Geometry: final body of the model. Coordinates: model frame, mm. A direction names the side the tool comes from. Give positions to 0.01 mm unless a question says otherwise; leave off trailing zeros. Order: outer loops, then holes, each group sorted by start corner. A loop starts at its lowest first (then second) coordinate and runs counter-clockwise, first axis right, second up. Notation, with made-up numbers: (-33, 63) - (-22, 63) arc R19 ccw to (-22, 68) - close; hole circle Ø4 at (-18.75, 35.25). An arc over 180 degrees is marked (long way). Put each result on its own line as item: value. Start each with the question number.
1. Mould query, pull axis Y, two halves, no side actions, for faces 1 (the flat face through (878.439, -338, 10)), 2 (the flat face through (672, -459.74, 10)), 3 (the flat face through (679, -254, 20.32)). Classes: pulls with the +Y half, pulls with the -Y half, needs draft (parallel to the pull), parting line crosses it, or undercut.
2. First-contact query: P1, Ø6, axis at x = 509, z = 14, coming from the +Y side. Flat tip, straight axial feed; report the tip coordinate or a pass-through.
3. Section C-C on x = 664.5. Return the cut outline in (y, z), plus the area to 3 significant figures.
4. Section B-B on z = 6. Count the separate pieces of the cut face and the enclosed holes in it, plus the area to 3 significant figures.
5. Set-up query: faces 4 (the flat face through (348, -44.45, 10)), 5 (the flat face through (508, -459.74, 10)), 6 (the flat face through (508, -54.61, 10)), 7 (the flat face through (878.439, -176, 10)), 8 (the flat face through (348, -469.9, 10)). Return all of +Z, -Z, +X, -X, +Y, -Y with unobstructed straight access to the full face (end or side cutting, diameter ignored); none if empty.
6. Ray query, line 1 along X through (y, z) = (-173, 10.5); line 2 along Y through (x, z) = (810.5, 18). Return the intervals inside material, ascending. Write a range as from..to.
7. Section A-A on y = -326. Return the cut outline in (x, z), plus the area to 3 significant figures.
from build123d import *

# Parameters (mm, degrees)
BOSS_EXTRUDE1_DEPTH = 20.32
SKETCH2_W           = 10.166490401
SKETCH2_H           = 81.316938585
SKETCH2_W_2         = 10.166490402
SKETCH2_H_2         = 81.316938584
SKETCH2_W_3         = 82.271298803
SKETCH2_H_3         = 10.16
CUT_EXTRUDE2_DEPTH  = 137.414
CUT_EXTRUDE3_DEPTH  = 1426.288377921
SKETCH5_W           = 82.296
SKETCH5_H           = 10.16
CUT_EXTRUDE4_DEPTH  = 1408.889980636
CUT_EXTRUDE5_DEPTH  = 1408.889980636
SKETCH7_W           = 370.520147136
SKETCH7_H           = 597.78628448
SKETCH7_W_2         = 231.394598612
SKETCH7_H_2         = 493.59842382
CUT_EXTRUDE6_DEPTH  = 25.4


with BuildPart() as part:
    # Sketch1 → Boss-Extrude1 (new body)
    with BuildSketch(Plane.XY):
        with BuildLine():
            Line((0, 0), (1345.447057269, 0))
            Line((1345.447057269, 0), (1156.937235756, -454.288839135))
            add(Edge.make_bspline(
                [(1156.937235756, -454.288839135), (1155.965204773, -456.631331547), (1154.630956054, -458.816896883), (1152.225947859, -461.69350105), (1151.355065983, -462.590813772), (1149.473312624, -464.260936999), (1148.45987476, -465.033112958), (1146.360299176, -466.401155283), (1145.26635201, -467.004685932), (1142.990856866, -468.052074807), (1141.798989191, -468.498505895), (1138.174492983, -469.560599459), (1135.699262078, -469.911644948), (1133.16419506, -469.9)],
                knots=[0, 0, 0, 0, 0.25, 0.25, 0.375, 0.375, 0.5, 0.5, 0.625, 0.625, 0.75, 0.75, 1, 1, 1, 1], degree=3))
            Line((1133.16419506, -469.9), (212.282862208, -469.9))
            add(Edge.make_bspline(
                [(188.509821513, -454.288839135), (189.481852496, -456.631331547), (190.816101215, -458.816896883), (193.22110941, -461.69350105), (194.091991286, -462.590813772), (195.973744645, -464.260936999), (196.987182509, -465.033112958), (199.086758093, -466.401155283), (200.180705259, -467.004685932), (202.456200403, -468.052074807), (203.648068078, -468.498505895), (207.272564286, -469.560599459), (209.747795191, -469.911644948), (212.282862208, -469.9)],
                knots=[0, 0, 0, 0, 0.25, 0.25, 0.375, 0.375, 0.5, 0.5, 0.625, 0.625, 0.75, 0.75, 1, 1, 1, 1], degree=3))
            Line((188.509821513, -454.288839135), (0, 0))
        make_face()
    extrude(amount=BOSS_EXTRUDE1_DEPTH)

    # Sketch2 → Cut-Extrude2 (cut)
    with BuildSketch(Plane.XY.offset(20.32)):
        with Locations((461.924984631, -337.764592123)):
            Rectangle(SKETCH2_W, SKETCH2_H)
        with Locations((883.522072638, -337.764592123)):
            Rectangle(SKETCH2_W_2, SKETCH2_H)
        with Locations((883.522072638, -175.130714953)):
            Rectangle(SKETCH2_W_2, SKETCH2_H_2)
        with Locations((461.924984631, -175.130714953)):
            Rectangle(SKETCH2_W, SKETCH2_H_2)
        with Locations((837.303178036, -464.82)):
            Rectangle(SKETCH2_W_3, SKETCH2_H_3)
        with Locations((672.723528635, -464.82)):
            Rectangle(SKETCH2_W_3, SKETCH2_H_3)
        with Locations((508.143879233, -464.82)):
            Rectangle(SKETCH2_W_3, SKETCH2_H_3)
    extrude(amount=-CUT_EXTRUDE2_DEPTH, mode=Mode.SUBTRACT)

    # Sketch4 → Cut-Extrude3 (cut, through all)
    with BuildSketch(Plane.XY.offset(20.32)):
        Polygon((0, 0), (1345.447057269, 0), (1327.002268746, -44.45), (18.444788523, -44.45), align=None)
    extrude(amount=-CUT_EXTRUDE3_DEPTH, mode=Mode.SUBTRACT)

    # Sketch5 → Cut-Extrude4 (cut, through all)
    with BuildSketch(Plane.XY.offset(20.32)):
        with Locations((508.131528634, -49.53)):
            Rectangle(SKETCH5_W, SKETCH5_H)
        with Locations((672.723528634, -49.53)):
            Rectangle(SKETCH5_W, SKETCH5_H)
        with Locations((837.315528634, -49.53)):
            Rectangle(SKETCH5_W, SKETCH5_H)
    extrude(amount=-CUT_EXTRUDE4_DEPTH, mode=Mode.SUBTRACT)

    # Sketch6 → Cut-Extrude5 (cut, through all)
    with BuildSketch(Plane.XY.offset(20.32)):
        Polygon((192.807539001, -448.077869782), (224.982862208, -469.9), (232.080223429, -549.766419732), (-59.510742861, -242.335130221), (-120.238907144, 37.382474964), (56.544788523, -44.45), (56.544788523, -119.698975594), align=None)
        Polygon((1120.46419506, -469.9), (1113.36683384, -549.766419732), (1404.95780013, -242.335130221), (1465.685964413, 37.382474964), (1288.902268746, -44.45), (1288.902268746, -119.698975594), (1152.639518267, -448.077869782), align=None)
    extrude(amount=-CUT_EXTRUDE5_DEPTH, mode=Mode.SUBTRACT)

    # Sketch7 → Cut-Extrude6 (cut)
    with BuildSketch(Plane.XY.offset(20.32)):
        with Locations((39.72278864, -171.00685776)):
            Rectangle(SKETCH7_W, SKETCH7_H)
        with Locations((1236.161494366, -223.10078809)):
            Rectangle(SKETCH7_W_2, SKETCH7_H_2)
    extrude(amount=-CUT_EXTRUDE6_DEPTH, mode=Mode.SUBTRACT)


solid = part.part
Resolved:
1. face 1: undercut
1. face 2: pulls with the -Y half
1. face 3: needs draft
2. P1: y = -54.61
3. outline: (-459.74, 0) - (-54.61, 0) - (-54.61, 20.32) - (-459.74, 20.32) - close
3. area: 8,230 mm^2
4. separate pieces: 1
4. enclosed holes: 4
4. area: 373,000 mm^2
5. face 4: +Z, -Z, +X, -X, +Y
5. face 5: +Z, -Z, -Y
5. face 6: +Z, -Z, +Y
5. face 7: +Z, -Z
5. face 8: +Z, -Z, +X, -X, -Y
6. line 1: 224.98..456.84, 467.01..878.44, 888.61..1120.46
6. line 2: -459.74..-54.61
7. outline: (224.98, 0) - (456.84, 0) - (456.84, 20.32) - (224.98, 20.32) - close; (467.01, 0) - (878.44, 0) - (878.44, 20.32) - (467.01, 20.32) - close; (888.61, 0) - (1120.46, 0) - (1120.46, 20.32) - (888.61, 20.32) - close
7. area: 17,800 mm^2
